from build123d import *

# Parameters (mm, degrees)
F0_W     = 876.3
F0_H     = 692.15
F1_DEPTH = 19.05
F2_R     = 3.175
F4_D     = 8.001
F4_DEPTH = 25.4
F4_TIP   = 2.4037429064
F6_D     = 8.001
F6_DEPTH = 25.4
F6_TIP   = 2.4037429064
F8_D     = 8.001
F8_DEPTH = 25.4
F8_TIP   = 2.4037429064


with BuildPart() as f1:
    # F0 (on Top) → F1 (new body)
    with BuildSketch(Plane.XY):
        Rectangle(F0_W, F0_H)
    extrude(amount=F1_DEPTH)

    # F2
    f2_edges = [f1.edges().sort_by_distance(p)[0] for p in [
        (0, -346.075, 19.05),
        (0, -346.075, 0),
    ]]
    fillet(f2_edges, radius=F2_R)

    # F4
    with Locations(Plane.YZ.offset(438.15)):
        with Locations((307.975, 9.525), (179.97424, 9.525), (51.97348, 9.525), (-76.02728, 9.525), (-204.02804, 9.525), (-300.02734, 9.525)):
            Hole(F4_D / 2, depth=F4_DEPTH)
            with Locations((0, 0, -(F4_DEPTH + F4_TIP / 2))):  # 118° drill point
                Cone(0, F4_D / 2, F4_TIP, mode=Mode.SUBTRACT)

    # F6
    with Locations(Plane(origin=(-438.15, 0, 0), x_dir=(0, -1, 0), z_dir=(-1, 0, 0))):
        with Locations((-307.975, 9.525), (-179.97424, 9.525), (-51.97348, 9.525), (76.02728, 9.525), (204.02804, 9.525), (300.02734, 9.525)):
            Hole(F6_D / 2, depth=F6_DEPTH)
            with Locations((0, 0, -(F6_DEPTH + F6_TIP / 2))):  # 118° drill point
                Cone(0, F6_D / 2, F6_TIP, mode=Mode.SUBTRACT)

    # F8
    with Locations(Plane(origin=(0, 346.075, 0), x_dir=(-1, 0, 0), z_dir=(0, 1, 0))):
        with Locations((-400.05, 9.525), (-272.04924, 9.525), (-144.04848, 9.525), (16.04772, 9.525), (144.04848, 9.525), (272.04924, 9.525), (400.05, 9.525)):
            Hole(F8_D / 2, depth=F8_DEPTH)
            with Locations((0, 0, -(F8_DEPTH + F8_TIP / 2))):  # 118° drill point
                Cone(0, F8_D / 2, F8_TIP, mode=Mode.SUBTRACT)


solid = f1.part
Verification items for the finished model (mm, model axes). Give positions to 0.01 mm unless a question says otherwise; leave off trailing zeros. Use CSV: the item, a comma, the result in double quotes.
1) Release check for a two-part mould opening along Z. For faces 1 (the face through (-6, 6, 19.05)), 2 (the face through (-6, 6, 0)), 3 (the face through (-438.15, -5, 9)) record: released by +Z, released by -Z, zero draft, split by the parting line, or undercut.
Final values:
face 1,"released by +Z"
face 2,"released by -Z"
face 3,"zero draft"
2) Go/stop test with flat-tipped pins: pin 1 Ø6.5 at (y, z) = (-300.03, 9.52) entering from -X; pin 2 Ø7 at (y, z) = (-76.03, 9.52) entering from -X; pin 3 Ø5 at (y, z) = (51.97, 9.52) entering from -X. Record where each tip stops, or that it passes through.
Final values:
pin 1,"x = -412.3"
pin 2,"x = -412.45"
pin 3,"x = -411.85"
3) Material ranges on line 1 along Z through (x, y) = (-400.05, 338); line 2 along Y through (x, z) = (100, 3) (3 decimals); line 3 along Y through (x, z) = (-272, 8.75) (3 decimals), recorded low to high.
Final values:
line 1,"0 to 5.52, 13.53 to 19.05"
line 2,"-346.07 to 346.075"
line 3,"-346.075 to 318.738"
